Part model, mm, in its own coordinate system. Round coordinates to 2 decimals unless told otherwise and drop trailing zeros. Write each loop counter-clockwise with the first axis right and the second up, starting at its lowest first coordinate (ties: lowest second). Pieces come first, ordered by that corner, then holes.
from build123d import *

# Parameters (mm, degrees)
BOSS_EXTRUDE1_DEPTH     = 88.9
CUT_EXTRUDE1_DEPTH      = 91.02678768
CUT_EXTRUDE1_DEPTH_BACK = 91.02678768
SKETCH3_R               = 2


with BuildPart() as part:
    # Sketch2 → Boss-Extrude1 (new, symmetric)
    with BuildSketch(Plane.XY):
        Polygon((-6.35, 6.35), (-6.35, -6.35), (6.35, -6.35), (6.35, 6.35), (3.175, 6.35), (3.175, -3.175), (-3.175, -3.175), (-3.175, 6.35), align=None)
    extrude(amount=BOSS_EXTRUDE1_DEPTH, both=True)

    # Sketch3 → Cut-Extrude1 (cut, two sides: drawn at the far end of the back side and taken through both)
    with BuildSketch(Plane(origin=(6.35, 0, 0), x_dir=(0, 0, -1), z_dir=(1, 0, 0)).offset(-CUT_EXTRUDE1_DEPTH_BACK)):
        with Locations(Location((-25.4, 0, 0), (0, 0, 90))):
            Circle(SKETCH3_R)
        with Locations(Location((76.2, 0, 0), (0, 0, 90))):
            Circle(SKETCH3_R)
        with BuildLine():
            Line((-82.55, 2), (-70.55, 2))
            ThreePointArc((-70.55, 2), (-68.55, 0), (-70.55, -2))
            Line((-70.55, -2), (-82.55, -2))
            ThreePointArc((-82.55, -2), (-84.55, 0), (-82.55, 2))
        make_face()
    extrude(amount=CUT_EXTRUDE1_DEPTH + CUT_EXTRUDE1_DEPTH_BACK, mode=Mode.SUBTRACT)


solid = part.part
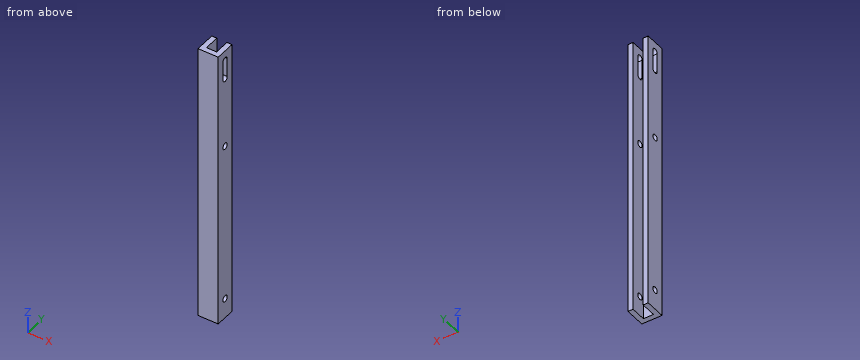
Q1. Saw through at C-C, the plane z = 15. Write the cut outline in (x, y) (3 decimals), and give its area (3 significant figures).
Q2. Wall check: line 1 (Z direction, x = -4.5, y = 0); line 2 (Y direction, x = -5.55, z = 25.4); line 3 (X direction, y = 3.25, z = -25) (3 decimals). Give the ranges that are in metal, low to high.
Q3. Saw through at D-D, the plane x = -1. Write the cut outline in (y, z) (3 decimals), and give its area (3 significant figures).
Q4. Drop a flat-ended pin along its axis: P1, Ø4, axis at x = -2.5, z = 9, coming from the +Y side. Give the stop position or say it passes through.
Q5. Saw through at A-A, the plane z = -76.2. Write the cut outline in (x, y) (3 decimals).
Q6. Saw through at B-B, the plane y = 0. Give the number of separate pieces and of enclosed holes in the cut face, and give its area (3 significant figures).
Computed:
1. outline: (-6.35, -6.35) - (6.35, -6.35) - (6.35, 6.35) - (3.175, 6.35) - (3.175, -3.175) - (-3.175, -3.175) - (-3.175, 6.35) - (-6.35, 6.35) - close
1. area: 101 mm2
2. line 1: z = -88.9 to -78.2, -74.2 to 23.4, 27.4 to 68.55, 84.55 to 88.9
2. line 2: y = -6.35 to -2, 2 to 6.35
2. line 3: x = -6.35 to -3.175, 3.175 to 6.35
3. outline: (-6.35, -88.9) - (-3.175, -88.9) - (-3.175, 88.9) - (-6.35, 88.9) - close
3. area: 565 mm2
4. P1: stops at y = 6.35
5. outline: (-6.35, -6.35) - (6.35, -6.35) - (6.35, -2) - (3.175, -2) - (3.175, -3.175) - (-3.175, -3.175) - (-3.175, -2) - (-6.35, -2) - close; (-6.35, 2) - (-3.175, 2) - (-3.175, 6.35) - (-6.35, 6.35) - close; (3.175, 2) - (6.35, 2) - (6.35, 6.35) - (3.175, 6.35) - close
6. separate pieces: 8
6. enclosed holes: 0
6. area: 977 mm2
